Design review of the part built by this model. Coordinates are the model's own, in mm. A direction names the side the tool comes from. Give positions to 0.01 mm unless a question says otherwise; leave off trailing zeros. Order: outer loops, then holes, each group sorted by start corner. A loop starts at its lowest first (then second) coordinate and runs counter-clockwise, first axis right, second up.
```python
from build123d import *

# Parameters (mm, degrees)
SKETCH1_W           = 36.83
SKETCH1_H           = 12.7
BOSS_EXTRUDE1_DEPTH = 50.8
SKETCH3_R           = 5.55625
CUT_EXTRUDE1_DEPTH  = 12.7


with BuildPart() as part:
    # Sketch1 → Boss-Extrude1 (new body)
    with BuildSketch(Plane.XY):
        Rectangle(SKETCH1_W, SKETCH1_H)
    extrude(amount=BOSS_EXTRUDE1_DEPTH)

    # Sketch3 → Cut-Extrude1 (cut)
    with BuildSketch(Plane.XY):
        with Locations((0, 6.35)):
            Circle(SKETCH3_R)
    extrude(amount=CUT_EXTRUDE1_DEPTH, mode=Mode.SUBTRACT)


solid = part.part
```
1. Take a section at B-B (x = 0). State the section outline as (y, z) points, then the cut area to 3 significant figures.
Recorded:
outline: (-6.35, 0) - (0.79, 0) - (0.79, 12.7) - (6.35, 12.7) - (6.35, 50.8) - (-6.35, 50.8) - close
area: 575 mm2
2. For line 1 along Z through (x, y) = (2.5, 2.25); line 2 along Y through (x, z) = (-0.5, 7); line 3 along Y through (x, z) = (1, 8.5), list the stretches that pass through material, from the lowest coordinate up.
Recorded:
line 1: z = 12.7 to 50.8
line 2: y = -6.35 to 0.82
line 3: y = -6.35 to 0.88
3. Draft analysis for pull direction X (two halves, no side actions). For faces 3 (the face through (0, 0, 50.8)), 4 (the face through (0, 4, 12.7)), 5 (the face through (18.415, 0, 25)), 6 (the face through (-18.415, 0, 25)), state which applies: pulls with the +X half, pulls with the -X half, needs draft (parallel to the pull), parting line crosses it, or undercut.
Recorded:
face 3: needs draft
face 4: undercut
face 5: pulls with the +X half
face 6: pulls with the -X half
4. Machinability: for faces 1 (the face through (0, 6.35, 25)), 2 (the face through (-0.122, 0.795, 6.261)), which of the approach directions +Z, -Z, +X, -X, +Y, -Y give a long, thin tool a straight path to every point of the face, cutting with its end or side? Answer none if there is none.
Recorded:
face 1: +Z, -Z, +X, -X, +Y
face 2: -Z, +Y
5. For pin 1 (1.7 mm diameter, centred on x = 0.5, y = 3, fed in from -Z), flat-tipped, find the tip position at first contact; note if it passes through.
Recorded:
pin 1: stops at z = 12.7
